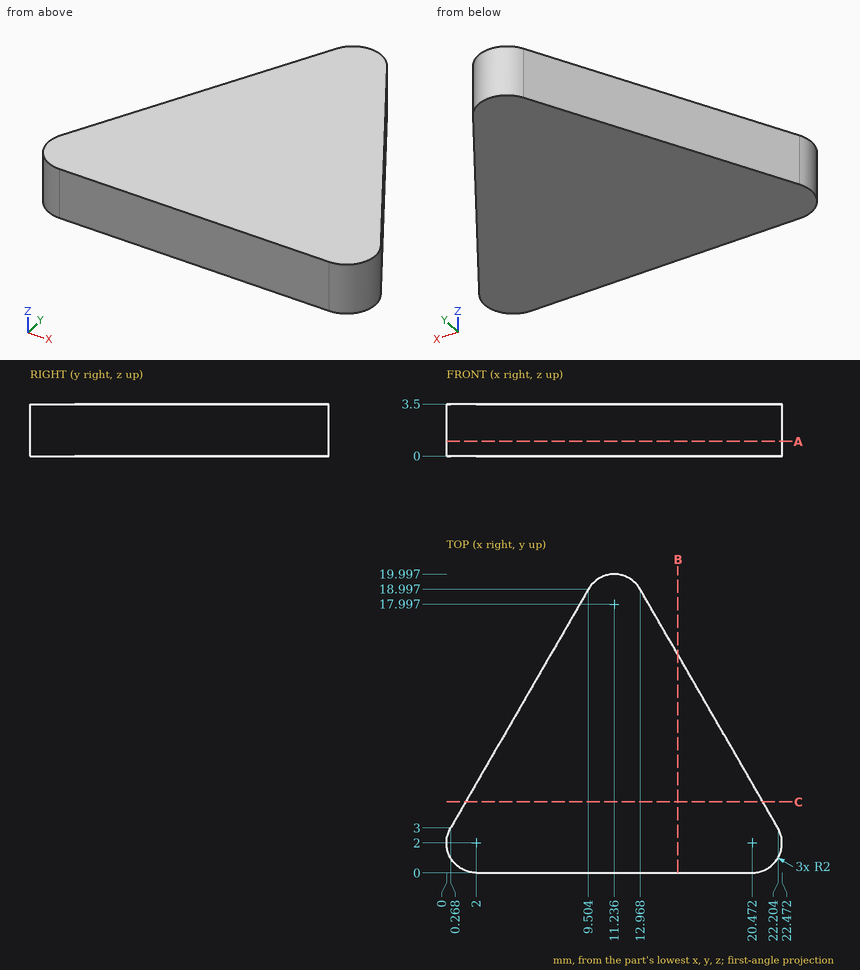
Geometry: see drawing. Coordinates: mm, zero at the bounding-box minimum. Give positions to 0.01 mm unless a question says otherwise; leave off trailing zeros. Loops run counter-clockwise (first coordinate to the right, second up) from the corner with the lowest first, then second, coordinate; pieces in that order, holes last. Notation, with made-up numbers: (40, -34.5) -> (96, -34.5) arc R33 cw to (96, -3.5) -> close; hole circle Ø7 at (34.5, 51). An arc over 180 degrees is marked (long way). Put each result on its own line as item: value.
1. Cut plane B-B (x = 15.5). Return the cut outline in (y, z).
Taken from the geometry:
outline: (0, 0) -> (14.61, 0) -> (14.61, 3.5) -> (0, 3.5) -> close
2. Cut plane C-C (y = 4.75). Return the cut outline in (x, z), plus the area to 3 significant figures.
Taken from the geometry:
outline: (1.28, 0) -> (21.19, 0) -> (21.19, 3.5) -> (1.28, 3.5) -> close
area: 69.7 mm2
3. Cut plane A-A (z = 1). Return the cut outline in (x, y).
Taken from the geometry:
outline: (0.27, 3) arc R2 ccw to (2, 0) -> (20.47, 0) arc R2 ccw to (22.2, 3) -> (12.97, 19) arc R2 ccw to (9.5, 19) -> close
4. Ray query, line 1 along X through (y, z) = (3.5, 0.7) (1 decimal); line 2 along Y through (x, z) = (21.5, 1.4) (1 decimal); line 3 along Y through (x, z) = (16.5, 3.1). Return the intervals inside material, ascending. Write a range as [from, to].
Taken from the geometry:
line 1: x = [0.6, 21.9]
line 2: y = [0.3, 4.2]
line 3: y = [0, 12.88]
5. Pin query (flat end, axial travel): P1, Ø1, axis at y = 15.5, z = 2, coming from the +X side. Return the tip coordinate at first contact, or that it passes through.
Taken from the geometry:
P1: stops at x = 15.28
